Work out the finished part from the listing and answer in its coordinate system (mm). Face numbers are marked on the shaded views. A direction names the side the tool comes from. Round coordinates to 2 decimals unless told otherwise and drop trailing zeros. Order: outer loops, then holes, each group sorted by start corner. A loop starts at its lowest first (then second) coordinate and runs counter-clockwise, first axis right, second up. Notation, with made-up numbers: M -26.5,20 L -10.5,20 A21 ccw -10.5,40 Z; hole C 79.5,69 d6. An arc over 180 degrees is marked long. Return JSON: item names as keys, results as strings.
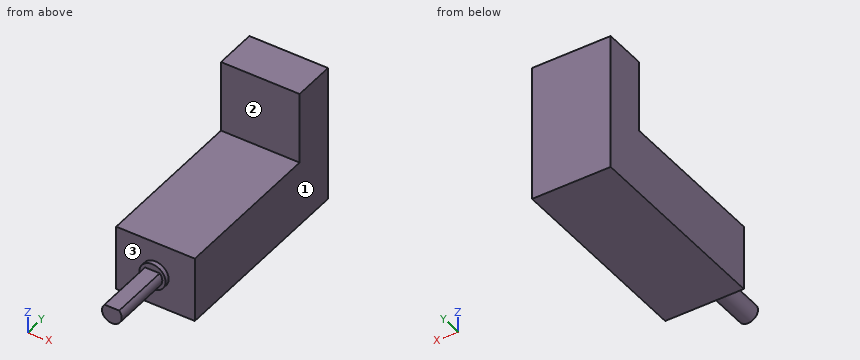
from build123d import *

# Parameters (mm, degrees)
F0_W     = 12
F0_H     = 10
F1_DEPTH = 30.5
F2_R     = 2
F3_DEPTH = 0.7
F4_R     = 1.5
F5_DEPTH = 9.3
F6_W     = 6.687609
F6_H     = 1.676586
F7_DEPTH = 9.3
F8_W     = 12
F8_H     = 6.5
F9_DEPTH = 11


with BuildPart() as f1:
    # F0 (on Front) → F1 (new body)
    with BuildSketch(Plane.XZ):
        Rectangle(F0_W, F0_H)
    extrude(amount=F1_DEPTH)

    # F2 (on face) → F3 (join)
    with BuildSketch(Plane.XZ.offset(30.5)):
        Circle(F2_R)
    extrude(amount=F3_DEPTH)

    # F4 (on face) → F5 (join)
    with BuildSketch(Plane.XZ.offset(31.2)):
        Circle(F4_R)
    extrude(amount=F5_DEPTH)

    # F6 (on face) → F7 (cut)
    with BuildSketch(Plane.XZ.offset(40.5)):
        with Locations((0.224422, 1.838293)):
            Rectangle(F6_W, F6_H)
    extrude(amount=-F7_DEPTH, mode=Mode.SUBTRACT)

    # F8 (on face) → F9 (join)
    with BuildSketch(Plane.XY.offset(5)):
        with Locations((0, -3.25)):
            Rectangle(F8_W, F8_H)
    extrude(amount=F9_DEPTH)


solid = f1.part
Item 1: Consider line 1 along Y through (x, z) = (0, -3.5); line 2 along Y through (x, z) = (-2, 11.75); line 3 along Z through (x, y) = (-4.5, -18). Determine where each line is inside the solid, lowest interval first. Write a range as [from, to].
Output:
{"line 1": "y = [-30.5, 0]", "line 2": "y = [-6.5, 0]", "line 3": "z = [-5, 5]"}
Item 2: Find section A-A (z = 0). Determine the outline of the cut face in (x, y), plus the area to 3 significant figures.
Output:
{"outline": "M -6,-30.5 L -2,-30.5 L -2,-31.2 L -1.5,-31.2 L -1.5,-40.5 L 1.5,-40.5 L 1.5,-31.2 L 2,-31.2 L 2,-30.5 L 6,-30.5 L 6,0 L -6,0 Z", "area": "397 mm^2"}
Item 3: Each of these flat-tipped pins is pushed along its axis until it touches: pin 1 (1.8 mm diameter, centred on x = 0, y = -38, fed in from +Z); pin 2 (3.5 mm diameter, centred on x = -0.5, y = -20, fed in from +Z). Where does it stop, or does it pass through?
Output:
{"pin 1": "stops at z = 1", "pin 2": "stops at z = 5"}
Item 4: Find section C-C (y = -23). Determine the outline of the cut face in (x, z).
Output:
{"outline": "M -6,-5 L 6,-5 L 6,5 L -6,5 Z"}
Item 5: Which of the six approach directions +Z, -Z, +X, -X, +Y, -Y give full straight-line access (tool end or side, diameter ignored) to the marked faces 1, 2 and 3?
Output:
{"face 1": "+Z, -Z, +X, +Y, -Y", "face 2": "+Z, +X, -X, -Y", "face 3": "-Y"}
Item 6: Find section B-B (x = 5.25). Determine the outline of the cut face in (y, z), plus the area to 4 significant figures.
Output:
{"outline": "M -30.5,-5 L 0,-5 L 0,16 L -6.5,16 L -6.5,5 L -30.5,5 Z", "area": "376.5 mm^2"}
Item 7: Find section D-D (x = 0). Determine the outline of the cut face in (y, z).
Output:
{"outline": "M -40.5,-1.5 L -31.2,-1.5 L -31.2,-2 L -30.5,-2 L -30.5,-5 L 0,-5 L 0,16 L -6.5,16 L -6.5,5 L -30.5,5 L -30.5,2 L -31.2,2 L -31.2,1 L -40.5,1 Z"}
